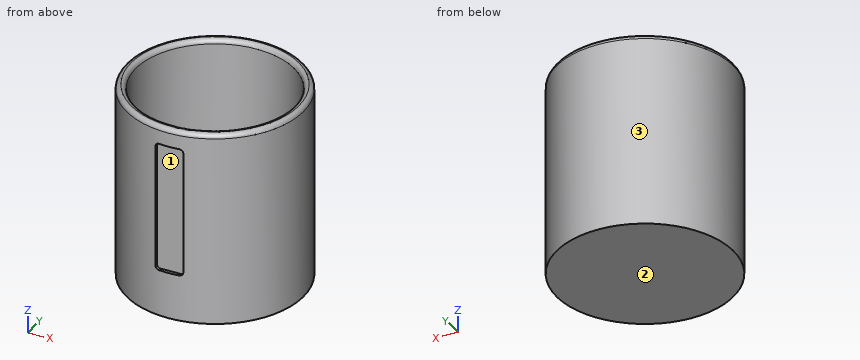
```python
from build123d import *

# Parameters (mm, degrees)
F0_R     = 47.5
F1_DEPTH = 5
F2_R     = 47.5
F2_R_2   = 42.5
F3_DEPTH = 100
F6_DEPTH = 2
F8_R     = 2.49999


# Not quite as in the source:
# - a fillet or chamfer is up to 0.001 mm smaller than in the source, because OpenCascade refuses the exact size


with BuildPart() as f1:
    # F0 (on Top) → F1 (new body)
    with BuildSketch(Plane.XY):
        Circle(F0_R)
    extrude(amount=F1_DEPTH)

    # F2 (on face) → F3 (join)
    with BuildSketch(Plane.XY.offset(5)):
        Circle(F2_R)
        Circle(F2_R_2, mode=Mode.SUBTRACT)
    extrude(amount=F3_DEPTH)

    # F5 (on offset) → F6 (cut)
    with BuildSketch(Plane.XZ.offset(47.5)):
        with BuildLine():
            ThreePointArc((7.5, 93), (6.9142135624, 94.4142135624), (5.5, 95))
            Line((5.5, 95), (-5.5, 95))
            ThreePointArc((-5.5, 95), (-6.9142135624, 94.4142135624), (-7.5, 93))
            Line((-7.5, 93), (-7.5, 27))
            ThreePointArc((-7.5, 27), (-6.9142135624, 25.5857864376), (-5.5, 25))
            Line((-5.5, 25), (5.5, 25))
            ThreePointArc((5.5, 25), (6.9142135624, 25.5857864376), (7.5, 27))
            Line((7.5, 27), (7.5, 93))
        make_face()
    extrude(amount=-F6_DEPTH, mode=Mode.SUBTRACT)

    # F8 (radius 2.5 in the source; OpenCascade refuses exactly that, so slightly less here)
    f8_edges = [f1.edges().sort_by_distance(p)[0] for p in [
        (-47.5, 0, 105),
        (-42.5, 0, 105),
    ]]
    fillet(f8_edges, radius=F8_R)


solid = f1.part
```
Can you work these out from the model? Positions are in its coordinate system, mm. Face numbers are marked on the shaded views. Give positions to 0.01 mm unless a question says otherwise; leave off trailing zeros. Write each loop counter-clockwise with the first axis right and the second up, starting at its lowest first coordinate (ties: lowest second). Pieces come first, ordered by that corner, then holes. Notation, with made-up numbers: (25.5, 69.5) -> (29.5, 69.5) arc R25 ccw to (29.5, 108.5) -> close; hole circle Ø4 at (-29.75, -14.75). An arc over 180 degrees is marked (long way). Write item = value, one per line.
(1) Suppose I cut it at D-D on z = 14.5. Write out the boundary of the cut face in (x, y).
Worked out:
outline = circle Ø95 at (0, 0); hole circle Ø85 at (0, 0)
(2) Suppose I cut it at C-C on z = 63.5. Write out the boundary of the cut face in (x, y).
Worked out:
outline = (-7.5, -46.9) -> (-7.5, -45.5) -> (7.5, -45.5) -> (7.5, -46.9) arc R47.5 ccw (long way) to start; hole circle Ø85 at (0, 0)
(3) I need wall thicknesses on probe 1 along Y at (x, z) = (0, 81); probe 2 along Z at (x, y) = (19.5, 4.5); probe 3 along Y at (x, z) = (-3, 55). Which ranges of each line are inside material? Lowest first, please. Write a range as from..to.
Worked out:
probe_1 = -45.5..-42.5, 42.5..47.5
probe_2 = 0..5
probe_3 = -45.5..-42.39, 42.39..47.41
(4) Thinking about a two-plate mould opening in X: for the marked faces 1, 2 and 3, which applies, released by +X, released by -X, zero draft, split by the parting line, or undercut?
Worked out:
face_1 = undercut
face_2 = zero draft
face_3 = split by the parting line
(5) I'm going to push flat-ended pins straight in: P1, Ø10, axis at x = 27.5, z = 20, coming from the -Y side; P2, Ø12, axis at y = -10.5, z = 20, coming from the +X side; P3, Ø5, axis at y = -15.5, z = 64.5, coming from the +X side. Where does each tip first touch, or does it pass through?
Worked out:
P1 = -41.83
P2 = 47.29
P3 = 45.69
